Could you check a few things on this drawing? It's one solid part, dimensions in mm from its lowest x, y, z. Give positions to 0.01 mm unless a question says otherwise; leave off trailing zeros. Write each loop counter-clockwise with the first axis right and the second up, starting at its lowest first coordinate (ties: lowest second). Pieces come first, ordered by that corner, then holes.
1. Suppose I cut it at A-A (z = 37.5). Please give me the cut outline in (x, y).
2. Suppose I cut it at C-C (y = 0.9). Give the number of separate pieces and of enclosed holes in the cut face, and give its area (3 significant figures).
3. If I drill on probe 1 along Z at (x, y) = (23.5, 1.3) (1 decimal); probe 2 along X at (y, z) = (1.4, 29.5) (1 decimal); probe 3 along Z at (x, y) = (74.5, 1.4) (1 decimal), over which ranges is the centre line in solid material (lowest first)?
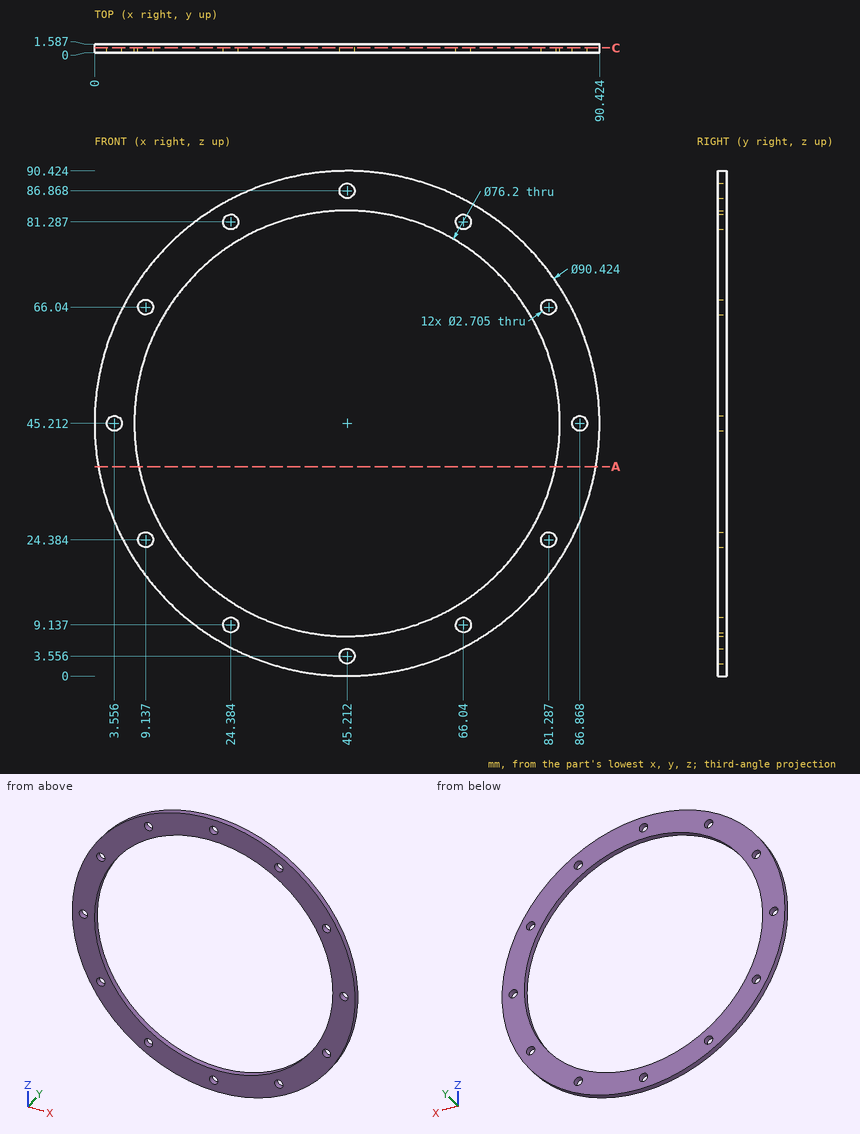
Checks:
1. outline: (0.66, 0) - (7.9, 0) - (7.9, 1.59) - (0.66, 1.59) - close; (82.52, 0) - (89.76, 0) - (89.76, 1.59) - (82.52, 1.59) - close
2. separate pieces: 1
2. enclosed holes: 13
2. area: 1,790 mm2
3. probe 1: z = 5.6 to 8.1, 10.2 to 13.9, 76.5 to 80.3, 82.3 to 84.9
3. probe 2: x = 2.8 to 10.5, 79.9 to 87.6
3. probe 3: z = 10.8 to 20.8, 69.6 to 79.7
